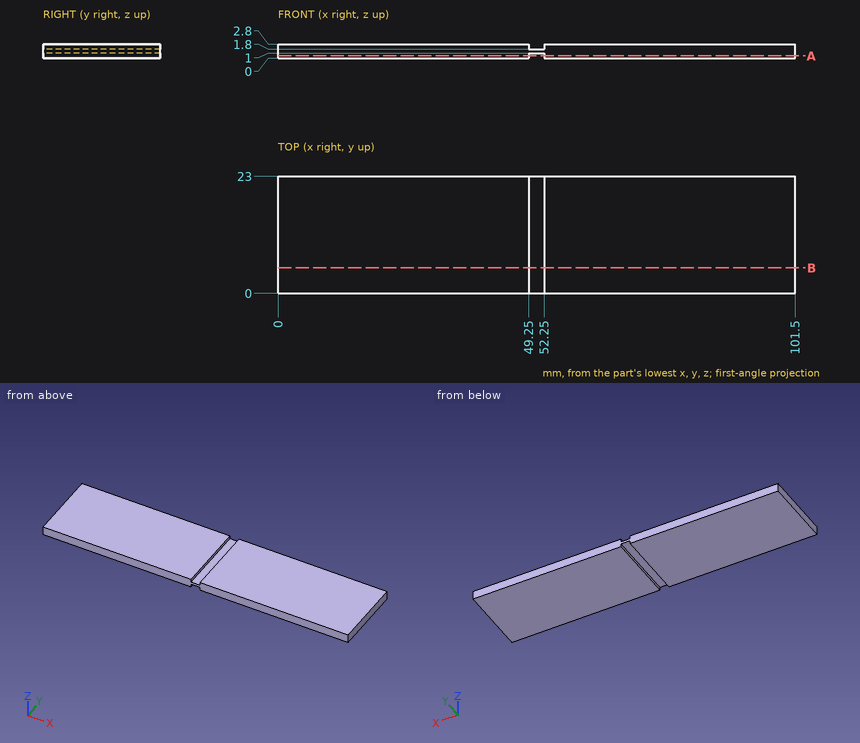
For this review, use the dimensioned drawing (mm, ordinates from the lowest corner) and the shaded views. Round coordinates to 2 decimals unless told otherwise and drop trailing zeros. Order: outer loops, then holes, each group sorted by start corner. A loop starts at its lowest first (then second) coordinate and runs counter-clockwise, first axis right, second up. Notation, with made-up numbers: M 33,-17 L 67,-17 A27 cw 67,17 Z; hole C 21,58 d8. An arc over 180 degrees is marked long. Use a Markdown table: item, result. Add a question column.
Item 1: Insertion check: pin 1 (1.5 mm diameter, centred on x = 51, y = 9, fed in from +Z). The pin has a flat end and moves straight along its axis. Give the tip position at first contact, or say it passes through.
Item 2: Add section B-B, the plane y = 5. Give the boundary of the cut face in (x, z), then the cut area to 3 significant figures.
Item 3: Add section A-A, the plane z = 0.45. Give the boundary of the cut face in (x, y), then the cut area to 3 significant figures.
Item 4: To check wall thickness, follow line 1 along X through (y, z) = (22, 2). State the ranges of the line that lie inside material, in increasing order.
Geometry results:
| question | item | result |
|---|---|---|
| 1 | pin 1 | stops at z = 1.8 |
| 2 | outline | M 0,0 L 49.25,0 L 49.25,1 L 52.25,1 L 52.25,0 L 101.5,0 L 101.5,2.8 L 52.25,2.8 L 52.25,1.8 L 49.25,1.8 L 49.25,2.8 L 0,2.8 Z |
| 2 | area | 278 mm² |
| 3 | outline | M 0,0 L 49.25,0 L 49.25,23 L 0,23 Z; M 52.25,0 L 101.5,0 L 101.5,23 L 52.25,23 Z |
| 3 | area | 2,270 mm² |
| 4 | line 1 | x = 0 to 49.25, 52.25 to 101.5 |
